For this review, take the finished solid that the model builds, in its own axes (mm). A direction names the side the tool comes from. Coordinates: 2 decimals unless noted, no trailing zeros. Loops run counter-clockwise (first coordinate to the right, second up) from the corner with the lowest first, then second, coordinate; pieces in that order, holes last. Notation, with made-up numbers: (75.25, 28) - (131.25, 28) arc R20 ccw to (131.25, 57) - close; hole circle Ø1 at (4, 22). An arc over 180 degrees is marked (long way). Answer as a JSON object with one key per item and string values. Group by question number.
Item 1: Mouldability with a two-part tool opening along Z and no side actions: class faces 1 (the flat face through (0, -15, -1)), 2 (the cylindrical face through (0.14, -4.436, -2.307)), 3 (the flat face through (-1, -15, 0)), 4 (the cylindrical face through (0, -25, 0)) as released by +Z, released by -Z, zero draft, split by the parting line, or undercut.
Item 2: Tool access review of faces 5 (the flat face through (1, -15, 0)), 6 (the flat face through (0, -15, 1)), 7 (the flat face through (10, 0, 0)): name each direction out of +Z, -Z, +X, -X, +Y, -Y from which nothing blocks a thin tool from reaching the whole face with its end or side.
Item 3: To check wall thickness, follow line 1 (X direction, y = -24, z = 0.5); line 2 (Y direction, x = -5.5, z = 2.25); line 3 (Z direction, x = -3.5, y = 1). State the ranges of each line that lie inside material, in increasing order.
Item 4: We need section D-D (x = -0.25). Give the boundary of the cut face in (y, z), then the cut area to 3 significant figures.
Item 5: We need section B-B (y = -10.5). Give the boundary of the cut face in (x, z), then the cut area to 3 significant figures.
Item 6: Clearance check with flat-ended pins moving along their axes: pin 1 (6 mm diameter, centred on y = -20, z = -2, fed in from -X); pin 2 (2 mm diameter, centred on x = 0, y = -10.5, fed in from -Z); pin 3 (2 mm diameter, centred on y = -13, z = 0, fed in from +X); pin 4 (4 mm diameter, centred on x = 4.5, y = -15.5, fed in from -Z). State where each tip first meets the part, or that it passes through.
Item 7: We need section C-C (x = 1.75). Give the boundary of the cut face in (y, z), then the cut area to 3 significant figures.
Item 8: We need section A-A (z = 0). Give the boundary of the cut face in (x, y).
from build123d import *

# Parameters (mm, degrees)
SKETCH1_R           = 5
BOSS_EXTRUDE1_DEPTH = 10
SKETCH2_W           = 2
SKETCH2_H           = 30
BOSS_EXTRUDE2_DEPTH = 1
SKETCH3_R           = 5
CUT_EXTRUDE1_DEPTH  = 33.341923258


with BuildPart() as part:
    # Sketch1 → Boss-Extrude1 (new, symmetric)
    with BuildSketch(Plane(origin=(0, 0, 0), x_dir=(0, 0, -1), z_dir=(1, 0, 0))):
        Circle(SKETCH1_R)
    extrude(amount=BOSS_EXTRUDE1_DEPTH, both=True)

    # Sketch2 → Boss-Extrude2 (add, symmetric)
    with BuildSketch(Plane.XY):
        with Locations((0, -15)):
            Rectangle(SKETCH2_W, SKETCH2_H)
    extrude(amount=BOSS_EXTRUDE2_DEPTH, both=True)

    # Sketch3 → Cut-Extrude1 (cut, through all)
    with BuildSketch(Plane(origin=(1, 0, 0), x_dir=(0, 0, -1), z_dir=(1, 0, 0))):
        with Locations((0, -30)):
            Circle(SKETCH3_R)
    extrude(amount=-CUT_EXTRUDE1_DEPTH, mode=Mode.SUBTRACT)


solid = part.part
Check sheet entries:
{
 "1": {"face 1": "released by -Z", "face 2": "split by the parting line", "face 3": "zero draft", "face 4": "undercut"},
 "2": {"face 5": "+Z, -Z, +X, -Y", "face 6": "+Z, +X, -X, -Y", "face 7": "+Z, -Z, +X, +Y, -Y"},
 "3": {"line 1": "x = -1 to 1", "line 2": "y = -4.47 to 4.47", "line 3": "z = -4.9 to 4.9"},
 "4": {"outline": "(-25.1, -1) - (-4.9, -1) arc R5 ccw (long way) to (-4.9, 1) - (-25.1, 1) arc R5 cw to start", "area": "119 mm2"},
 "5": {"outline": "(-1, -1) - (1, -1) - (1, 1) - (-1, 1) - close", "area": "4.00 mm2"},
 "6": {"pin 1": "stops at x = -1", "pin 2": "stops at z = -1", "pin 3": "stops at x = 1", "pin 4": "passes through"},
 "7": {"outline": "circle Ø10 at (0, 0)", "area": "78.5 mm2"},
 "8": {"outline": "(-10, -5) - (-1, -5) - (-1, -25) - (1, -25) - (1, -5) - (10, -5) - (10, 5) - (-10, 5) - close"}
}
